Solid Edge part; units mm, degrees
sketch "Sketch1" plane through (0, 0, 0) normal (1, 0, 0) x (0, 1, 0)
  circle A0 centre (0, 0) radius 5
extrude "Protrusion1" add sketch "Sketch1" along normal mid plane 69
sketch "Sketch2" plane through (24.5, 0, 0) normal (1, 0, 0) x (0, 1, 0)
  circle A0 centre (0, 0) radius 5
extrude "ExtrudedCutout_1" cut sketch "Sketch2" along normal blind 2
sketch "Sketch3" plane through (24.5, 0, 0) normal (1, 0, 0) x (0, 1, 0)
  circle A0 centre (0, 0) radius 3
extrude "ExtrudedProtrusion_4" add sketch "Sketch3" along normal blind 2
sketch "Sketch4" plane through (-29.5, 0, 0) normal (-1, 0, 0) x (0, -1, 0)
  circle A0 centre (0, 0) radius 5
extrude "ExtrudedCutout_2" cut sketch "Sketch4" along normal blind 1.5
sketch "Sketch5" plane through (-29.5, 0, 0) normal (-1, 0, 0) x (0, -1, 0)
  circle A0 centre (0, 0) radius 4
extrude "ExtrudedProtrusion_5" add sketch "Sketch5" along normal blind 1.5
chamfer "Chamfer_1" distance 0.5 angle 45 2 edges at (-34.5, -5, 0) (34.5, -5, 0) measured on face at (-34.5, 3.2333, -3.4333)
sketch "Sketch6" plane through (0, -3.2, 0) normal (0, -1, 0) x (1, 0, 0)
  line L0 (-34.5, -1.5) -> (-34.5, 1.5)
  line L1 (-34.5, 1.5) -> (-9, 1.5)
  arc A0 (-9, 1.5) -> (-9, -1.5) centre (-9, 0) cw
  line L2 (-9, -1.5) -> (-34.5, -1.5)
extrude "ExtrudedCutout_3" cut sketch "Sketch6" along normal blind 30
cosmetic_thread "Thread_5" thread depth 7
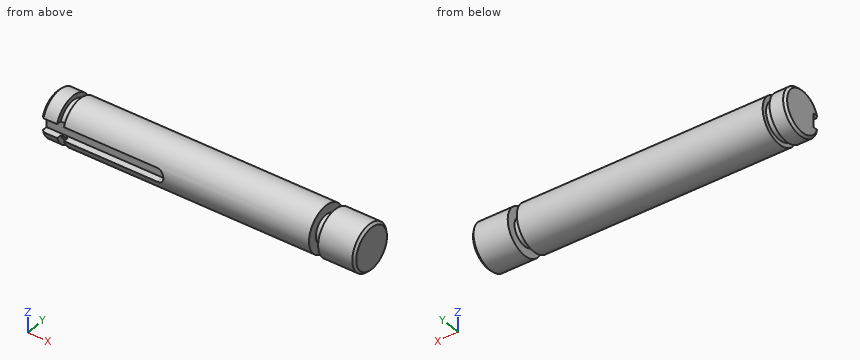
Geometry check sheet. Reference: the model listing, model coordinates, mm. Round coordinates to 2 decimals unless told otherwise and drop trailing zeros. Write each loop counter-clockwise with the first axis right and the second up, starting at its lowest first coordinate (ties: lowest second). Pieces come first, ordered by that corner, then holes. Notation, with made-up numbers: (54, -21) - (74, -21) arc R22 cw to (74, 12) - close; hole circle Ø11 at (-19, 71). An arc over 180 degrees is marked (long way). One line per item, written item: value.
1. Cross-section at B-B on z = 0. Record the boundary of the cut face in (x, y).
The answers:
outline: (-34.5, -3.2) - (-7.5, -3.2) - (-7.5, -5) - (24.5, -5) - (24.5, -3) - (26.5, -3) - (26.5, -5) - (34, -5) - (34.5, -4.5) - (34.5, 4.5) - (34, 5) - (26.5, 5) - (26.5, 3) - (24.5, 3) - (24.5, 5) - (-29.5, 5) - (-29.5, 4) - (-31, 4) - (-31, 5) - (-34, 5) - (-34.5, 4.5) - close
2. Cross-section at A-A on y = 0. Record the boundary of the cut face in (x, z).
The answers:
outline: (-34.5, -4.5) - (-34, -5) - (-31, -5) - (-31, -4) - (-29.5, -4) - (-29.5, -5) - (24.5, -5) - (24.5, -3) - (26.5, -3) - (26.5, -5) - (34, -5) - (34.5, -4.5) - (34.5, 4.5) - (34, 5) - (26.5, 5) - (26.5, 3) - (24.5, 3) - (24.5, 5) - (-29.5, 5) - (-29.5, 4) - (-31, 4) - (-31, 5) - (-34, 5) - (-34.5, 4.5) - close
3. Cross-section at C-C on x = 4.5. Record the boundary of the cut face in (y, z), and give its area (3 significant figures).
The answers:
outline: circle Ø10 at (0, 0)
area: 78.5 mm^2
4. Depth check by flat-ended pin: pin 1 Ø1.3 at (x, y) = (-23, -4) entering from -Z; pin 2 Ø1.7 at (x, y) = (-16.5, -4) entering from +Z; pin 3 Ø2.5 at (x, z) = (-14.5, 0) entering from -Y. Enter the tip coordinate at first touch or a pass-through.
The answers:
pin 1: stops at z = -3.71
pin 2: stops at z = 3.88
pin 3: stops at y = -3.2
5. Scan lines: L1, parallel to X at y = 1.75, z = -4; L2, parallel to X at y = 3, z = -1.75; L3, parallel to Z at x = 4.5, y = -0.25. Record each from-to range of solid material in increasing order.
The answers:
L1: x = -34.5 to -31, -29.5 to 24.5, 26.5 to 34.5
L2: x = -34.5 to 24.5, 26.5 to 34.5
L3: z = -4.99 to 4.99
6. Cross-section at D-D on x = -12.5. Record the boundary of the cut face in (y, z), and give its area (3 significant figures).
The answers:
outline: (-4.77, -1.5) arc R5 ccw (long way) to (-4.77, 1.5) - (-3.2, 1.5) - (-3.2, -1.5) - close
area: 73.4 mm^2
